Check sheet for the modelled part. Datum: model origin and axes. Units: mm. Give positions to 0.01 mm unless a question says otherwise; leave off trailing zeros. Write each loop counter-clockwise with the first axis right and the second up, starting at its lowest first coordinate (ties: lowest second). Pieces come first, ordered by that corner, then holes. Notation, with made-up numbers: (-37.5, 49) -> (-28.5, 49) arc R20 cw to (-28.5, 65) -> close; hole circle Ø10 at (24, 88.25). An arc over 180 degrees is marked (long way). Use a Markdown table: item, result. Add a question column.
1. Cross-section at A-A (x = 25). Enter the section's corners in (y, z).
2. Scan lines: probe 1 along X at (y, z) = (-47.5, 1.4); probe 2 along Y at (x, z) = (-74, 1.1); probe 3 along X at (y, z) = (-14.5, 1). Record each from-to range of solid material in increasing order. Write a range as [from, to].
3. Cross-section at B-B (y = 77.5). Enter the section's corners in (x, z), then the cut area to 3 significant figures.
4. Cross-section at C-C (x = -11). Enter the section's corners in (y, z), then the cut area to 3 significant figures.
5. Gauge pin test, flat ends, axial feed: P1, Ø1, axis at y = -34.5, z = 0.5, coming from the +X side; P2, Ø1.9, axis at x = -74.59, y = -31.63, coming from the -Z side; P3, Ø3, axis at x = -60, z = 1, coming from the -Y side. Record the tip position at first contact, or that the pin passes through.
6. Cross-section at D-D (z = 0.45). Count the separate pieces of the cut face and the enclosed holes in it, then the cut area to 3 significant figures.
from build123d import *
from OCP.BRepFilletAPI import BRepFilletAPI_MakeChamfer

# Parameters (mm, degrees)
SKETCH_1_R          = 2.1
EXTRUDE_1_DEPTH     = 2.5
CUT_EXTRUDE_1_DEPTH = 95.372930441
EXTRUDE_2_DEPTH     = 5
CUT_EXTRUDE_2_DEPTH = 142.00635371
FILLET_1_R          = 5
FILLET_2_R          = 4
FILLET_3_R          = 15
CHAMFER_1_SIZE      = 4
CHAMFER_1_SIZE2     = 6.20437999
CHAMFER_2_SIZE      = 2
SKETCH_6_R          = 3.1
CUT_EXTRUDE_3_DEPTH = 140.696602049
CUT_EXTRUDE_4_DEPTH = 140.696602049
SKETCH_8_R          = 1.55
CUT_EXTRUDE_5_DEPTH = 140.696602049
FILLET_4_R          = 1
CHAMFER_3_SIZE      = 3


with BuildPart() as part:
    # 草图1 → 凸台-拉伸1 (new, symmetric)
    with BuildSketch(Plane.XY):
        Polygon((-35, 87.5), (-35, -87.5), (35, -87.5), (35, -67.5), (-15, 87.5), align=None)
        with Locations((-25, -77.5)):
            Circle(SKETCH_1_R, mode=Mode.SUBTRACT)
        with Locations((25, -77.5)):
            Circle(SKETCH_1_R, mode=Mode.SUBTRACT)
        with Locations((-25, 77.5)):
            Circle(SKETCH_1_R, mode=Mode.SUBTRACT)
        with Locations((-25, -57.5)):
            Circle(SKETCH_1_R, mode=Mode.SUBTRACT)
    extrude(amount=EXTRUDE_1_DEPTH, both=True)

    # 草图2 → 切除-拉伸1 (cut, through all)
    with BuildSketch(Plane(origin=(0, 0, -2.5), x_dir=(-1, 0, 0), z_dir=(0, 0, -1))):
        with BuildLine():
            Line((-17.130804412, -60.9649861), (5.241456911, 8.389024))
            ThreePointArc((5.241456911, 8.389024), (11.5350139, 11.612553189), (14.758543089, 5.318996201))
            Line((14.758543089, 5.318996201), (-7.613718234, -64.0350139))
            ThreePointArc((-7.613718234, -64.0350139), (-13.907275222, -67.258543089), (-17.130804412, -60.9649861))
        make_face()
    extrude(amount=-CUT_EXTRUDE_1_DEPTH, mode=Mode.SUBTRACT)

    # 草图3 → 凸台-拉伸2 (add)
    with BuildSketch(Plane(origin=(0, 0, -2.5), x_dir=(-1, 0, 0), z_dir=(0, 0, -1))):
        Polygon((35, -87.5), (92.302946454, -84.303295451), (110.460589291, -75.918785529), (35, 87.5), align=None)
    extrude(amount=-EXTRUDE_2_DEPTH)

    # 草图5 → 切除-拉伸2 (cut, through all)
    with BuildSketch(Plane(origin=(0, 0, -2.5), x_dir=(-1, 0, 0), z_dir=(0, 0, -1))):
        Polygon((35, 39.792977913), (58.598142626, -11.311576727), (35, -65.049025296), align=None)
        Polygon((87.794289034, -74.539267276), (40.598003783, -77.172161204), (64.196146409, -23.434712635), align=None)
    extrude(amount=-CUT_EXTRUDE_2_DEPTH, mode=Mode.SUBTRACT)

    # 圆角1
    fillet_1_edges = [part.edges().sort_by_distance(p)[0] for p in [
        (-64.196146409, -23.434712635, 0),
        (-87.794289034, -74.539267276, 0),
        (-40.598003783, -77.172161204, 0),
        (-35, 39.792977913, 0),
    ]]
    fillet(fillet_1_edges, radius=FILLET_1_R)

    # 圆角2
    fillet_2_edges = [part.edges().sort_by_distance(p)[0] for p in [
        (-35, -65.049025296, 0),
    ]]
    fillet(fillet_2_edges, radius=FILLET_2_R)

    # 圆角3
    fillet_3_edges = [part.edges().sort_by_distance(p)[0] for p in [
        (-58.598142626, -11.311576727, 0),
    ]]
    fillet(fillet_3_edges, radius=FILLET_3_R)

    # 倒角1: one chamfer whose edges measure the first distance from different faces: ONE call of the kernel's chamfer builder (chamfer() names one face for all edges)
    chamfer_1_edges_1 = [part.edges().sort_by_distance(p)[0] for p in [
        (-110.460589291, -75.918785529, 0),
        (35, -87.5, 0),
    ]]
    chamfer_1_edges_2 = [part.edges().sort_by_distance(p)[0] for p in [
        (-15, 87.5, 0),
    ]]
    chamfer_1_side_2 = [part.faces().sort_by_distance(p)[0] for p in [
        (-25, 87.5, 0),
    ]]
    chamfer_1 = BRepFilletAPI_MakeChamfer(part.part.solid().wrapped)
    for e in chamfer_1_edges_1:
        chamfer_1.Add(CHAMFER_1_SIZE, e.wrapped)
    for e in chamfer_1_edges_2:
        chamfer_1.Add(CHAMFER_1_SIZE, CHAMFER_1_SIZE2, e.wrapped, chamfer_1_side_2[0].wrapped)  # the first distance lies on this face
    add(Compound.cast(chamfer_1.Shape()), mode=Mode.REPLACE)

    # 倒角2
    chamfer_2_edges = [part.edges().sort_by_distance(p)[0] for p in [
        (22.9, -77.5, -2.5),
        (-27.1, -77.5, -2.5),
        (-27.1, 77.5, -2.5),
        (-27.1, -57.5, -2.5),
    ]]
    chamfer(chamfer_2_edges, length=CHAMFER_2_SIZE)

    # 草图6 → 切除-拉伸3 (cut, through all)
    with BuildSketch(Plane(origin=(0, 0, -2.5), x_dir=(-1, 0, 0), z_dir=(0, 0, -1))):
        with Locations((97.189512912, -71.032219072)):
            Circle(SKETCH_6_R)
        with Locations((44.786325904, 42.453048657)):
            Circle(SKETCH_6_R)
    extrude(amount=-CUT_EXTRUDE_3_DEPTH, mode=Mode.SUBTRACT)

    # 草图7 → 切除-拉伸4 (cut, through all)
    with BuildSketch(Plane.XY.offset(2.5)):
        Polygon((-58.057402283, 37.566482199), (-53.170835826, 24.29540582), (-88.805002991, -52.874576235), (-102.07607937, -57.761142693), align=None)
    extrude(amount=-CUT_EXTRUDE_4_DEPTH, mode=Mode.SUBTRACT)

    # 草图8 → 切除-拉伸5 (cut, through all)
    with BuildSketch(Plane.XY.offset(2.5)):
        with Locations((-49.224888136, 23.299415443)):
            Circle(SKETCH_8_R)
        with Locations((-62.849716758, -6.206754167)):
            Circle(SKETCH_8_R)
        with Locations((-74.588030648, -31.627454138)):
            Circle(SKETCH_8_R)
        with Locations((-80.666800341, -44.791745195)):
            Circle(SKETCH_8_R)
    extrude(amount=-CUT_EXTRUDE_5_DEPTH, mode=Mode.SUBTRACT)

    # 圆角4
    fillet_4_edges = [part.edges().sort_by_distance(p)[0] for p in [
        (-53.170835826, 24.29540582, 0),
        (-88.805002991, -52.874576235, 0),
    ]]
    fillet(fillet_4_edges, radius=FILLET_4_R)

    # 倒角3
    chamfer_3_edges = [part.edges().sort_by_distance(p)[0] for p in [
        (-94.089512912, -71.032219072, 2.5),
        (-41.686325904, 42.453048657, 2.5),
    ]]
    chamfer(chamfer_3_edges, length=CHAMFER_3_SIZE)


solid = part.part
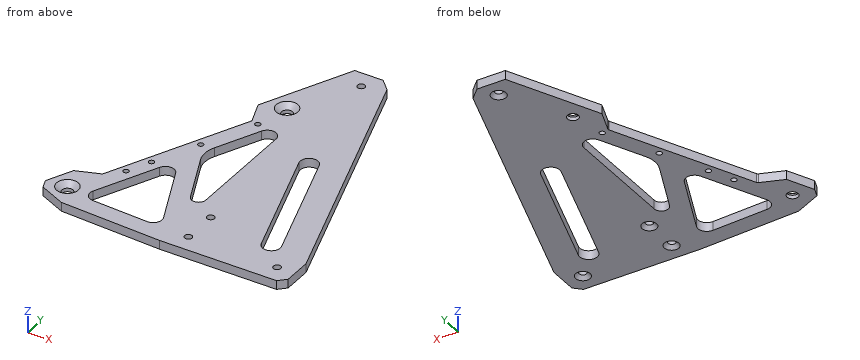
Worked answers:
| question | item | result |
|---|---|---|
| 1 | outline | (-87.5, -2.5) -> (-81.6, -2.5) -> (-79.6, -0.5) -> (-79.6, 2.5) -> (-87.5, 2.5) -> close; (-75.4, -0.5) -> (-73.4, -2.5) -> (-36.5, -2.5) -> (-36.5, 2.5) -> (-75.4, 2.5) -> close |
| 2 | probe 1 | x = [-86.32, -75.31], [-53.63, -42.71], [-35.3, 2.28], [12.79, 28.55] |
| 2 | probe 2 | y = [-85.32, -75.31], [-44.67, -33.06], [-30.19, -20.81] |
| 2 | probe 3 | x = [-71.09, -56.84], [-35, -8.37], [2.14, 17.9] |
| 3 | outline | (-39.62, -2.5) -> (-29.1, -2.5) -> (-27.1, -0.5) -> (-27.1, 2.5) -> (-39.62, 2.5) -> close; (-22.9, -0.5) -> (-20.9, -2.5) -> (-11.77, -2.5) -> (-11.77, 2.5) -> (-22.9, 2.5) -> close |
| 3 | area | 114 mm² |
| 4 | outline | (-87.5, -2.5) -> (-6.33, -2.5) -> (-6.33, 2.5) -> (-87.5, 2.5) -> close; (11.75, -2.5) -> (75.1, -2.5) -> (75.1, 2.5) -> (11.75, 2.5) -> close |
| 4 | area | 723 mm² |
| 5 | P1 | stops at x = 24.52 |
| 5 | P2 | passes through |
| 5 | P3 | stops at y = -86.19 |
| 6 | separate pieces | 1 |
| 6 | enclosed holes | 13 |
| 6 | area | 10,900 mm² |
